Work out the finished part from the listing and answer in its coordinate system (mm). Face numbers are marked on the shaded views. Give positions to 0.01 mm unless a question says otherwise; leave off trailing zeros. Loops run counter-clockwise (first coordinate to the right, second up) from the corner with the lowest first, then second, coordinate; pieces in that order, holes last. Notation, with made-up numbers: (-37.5, -7.75) - (-30.5, -7.75) arc R12 cw to (-30.5, -1.75) - close; hole circle Ø9 at (50.5, -23.5). An arc over 180 degrees is marked (long way). Use one line per item in the form item = value. Start each with the question number.
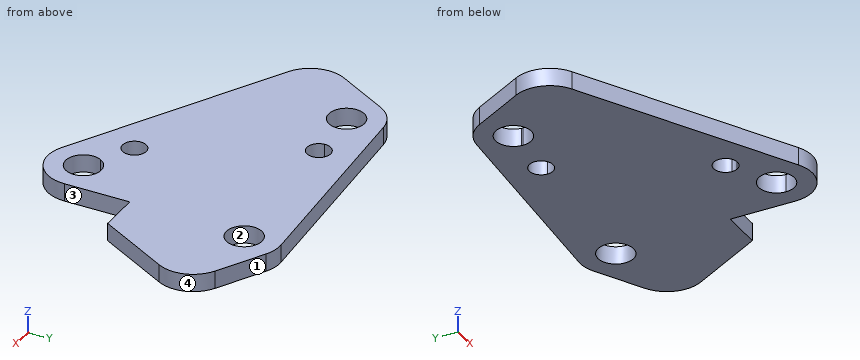
from build123d import *

# Parameters (mm, degrees)
F0_R     = 4.7625
F1_DEPTH = 4.7625


# Not quite as in the source:
# - a length typed as a fraction of an inch, garbled in the dataset ("3 / 203.2 mm" for 3/8 in), is restored


with BuildPart() as f1:
    # F0 (on Top) → F1 (new body)
    with BuildSketch(Plane.XY):
        with BuildLine():
            Line((-60.1561630362, 22.4546581751), (-4.6178116328, -8.3307527105))
            ThreePointArc((-4.6178116328, -8.3307527105), (4.8343029072, -8.2070177532), (9.525, 0))
            Line((9.525, 0), (9.525, 17.4625))
            Line((9.525, 17.4625), (20.5700693075, 17.4625))
            Line((20.5700693075, 17.4625), (31.4198108747, 37.0359519197))
            ThreePointArc((31.4198108747, 37.0359519197), (32.245075818, 44.2792093667), (27.7068697971, 49.984516263))
            Line((27.7068697971, 49.984516263), (15.2107407313, 56.9112337123))
            ThreePointArc((15.2107407313, 56.9112337123), (12.6684281132, 57.8766054007), (9.9569358455, 58.0842243475))
            Line((9.9569358455, 58.0842243475), (-48.4779919349, 54.1737420822))
            ThreePointArc((-48.4779919349, 54.1737420822), (-52.9477518555, 52.7109507654), (-56.1727513924, 49.2878103693))
            Line((-56.1727513924, 49.2878103693), (-63.8691041139, 35.4032225185))
            ThreePointArc((-63.8691041139, 35.4032225185), (-64.6943690572, 28.1599650715), (-60.1561630362, 22.4546581751))
        make_face()
        with BuildLine():
            ThreePointArc((-9.3211290658, 6.9267174493), (-9.4222603076, 6.1317609364), (-9.7192114956, 5.387446905))
            ThreePointArc((-9.7192114956, 5.387446905), (-15.569997824, 7.7216739621), (-9.3211290658, 6.9267174493))
        make_face(mode=Mode.SUBTRACT)
        with BuildLine():
            ThreePointArc((4.7625, 0), (-1.1924347693, -4.6108031373), (-4.1653763553, 2.3089058164))
            ThreePointArc((-4.1653763553, 2.3089058164), (1.1924347693, 4.6108031373), (4.7625, 0))
        make_face(mode=Mode.SUBTRACT)
        with BuildLine():
            ThreePointArc((-43.0794986819, 44.6699987365), (-52.6018408585, 44.510911641), (-43.0901270091, 44.987995363))
            ThreePointArc((-43.0901270091, 44.987995363), (-43.0821565054, 44.829085832), (-43.0794986819, 44.6699987365))
        make_face(mode=Mode.SUBTRACT)
        with BuildLine():
            ThreePointArc((-28.827426439, 45.7299874915), (-31.8963683753, 42.5567593737), (-35.1703408876, 45.5179897405))
            ThreePointArc((-35.1703408876, 45.5179897405), (-32.1084845027, 48.9032156092), (-28.827426439, 45.7299874915))
        make_face(mode=Mode.SUBTRACT)
        with Locations((10.5929290985, 48.5804810018)):
            Circle(F0_R, mode=Mode.SUBTRACT)
    extrude(amount=F1_DEPTH)


solid = f1.part
1) A cutting plane is placed at C-C (z = 3.75). State how many separate pieces and enclosed holes the cut face has, plus the area to 3 significant figures.
2) A cutting plane is placed at D-D (x = -20). Give the vertices of the cut face in (y, z), plus the area to 3 significant figures.
3) A cutting plane is placed at B-B (x = -47.5). Give the vertices of the cut face in (y, z).
4) Flat-ended cylindrical pins translate along their axes: pin 1 Ø10 at (x, y) = (-12.5, 6.93) entering from -Z; pin 2 Ø1 at (x, z) = (-54.5, 3) entering from -Y; pin 3 Ø2.5 at (y, z) = (7, 3.5) entering from +X (3 decimals). Find the tip coordinate at first contact, or state that the pin passes through.
5) A cutting plane is placed at A-A (y = -3). Give the vertices of the cut face in (x, z).
6) Find the intervals of material crossed by probe 1 along X at (y, z) = (45, 0.2); probe 2 along Y at (x, z) = (-48, 2.95); probe 3 along Y at (x, z) = (-47, 3.6), in increasing order.
7) Determine the mould class of the marked faces 1, 2, 3 and 4 for opening direction Y: released by +Y, released by -Y, zero draft, split by the parting line, or undercut.
Answer sheet:
q1.separate_pieces = 1
q1.enclosed_holes = 5
q1.area = 4,040 mm²
q2.outline = (0.2, 0) - (56.08, 0) - (56.08, 4.76) - (0.2, 4.76) - close
q2.area = 266 mm²
q3.outline = (15.44, 0) - (39.92, 0) - (39.92, 4.76) - (15.44, 4.76) - close; (49.42, 0) - (54.24, 0) - (54.24, 4.76) - (49.42, 4.76) - close
q4.pin_1 = 0
q4.pin_2 = 19.04
q4.pin_3 = 9.525
q5.outline = (-14.23, 0) - (-3.7, 0) - (-3.7, 4.76) - (-14.23, 4.76) - close; (3.7, 0) - (9.04, 0) - (9.04, 4.76) - (3.7, 4.76) - close
q6.probe_1 = -58.55 to -52.59, -43.09 to -35.09, -28.91 to 7.45, 13.73 to 32.01
q6.probe_2 = 15.72 to 39.91, 49.43 to 54.21
q6.probe_3 = 15.16 to 39.98, 49.36 to 54.27
q7.face_1 = released by +Y
q7.face_2 = undercut
q7.face_3 = zero draft
q7.face_4 = split by the parting line
